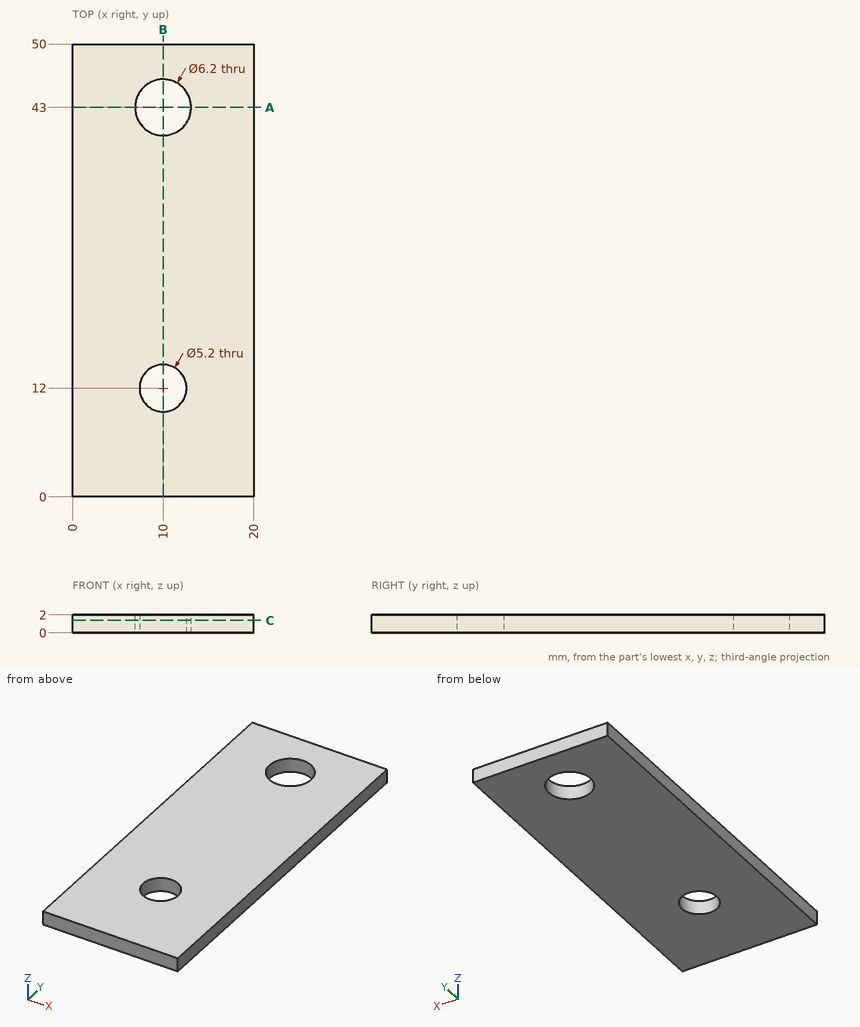
Study the drawing (mm; zero at the part's minimum x, y, z) and answer. Coordinates: 2 decimals unless noted, no trailing zeros. Loops run counter-clockwise (first coordinate to the right, second up) from the corner with the lowest first, then second, coordinate; pieces in that order, holes last. Notation, with made-up numbers: M -31.5,35 L 2.5,35 A22 cw 2.5,70 Z; hole C 54.5,24.25 d11. An arc over 180 degrees is marked long. Answer in a Markdown table with one row per item. Add a question column.
1. Consider L1, parallel to Y at x = 10, z = 0.5; L2, parallel to Y at x = 11.5, z = 0.2; L3, parallel to X at y = 42.5, z = 0.15. Determine where each line is inside the solid, lowest interval first.
2. A flat-ended cylindrical pin translates along its axis: P1, Ø5, axis at x = 10, y = 43, coming from the +Z side. Find the tip coordinate at first contact, or state that the pin passes through.
3. Find section C-C, the plane z = 1.4. Write down the section's boundary in (x, y).
4. Find section A-A, the plane y = 43. Write down the section's boundary in (x, z), then the cut area to 3 significant figures.
5. Find section B-B, the plane x = 10. Write down the section's boundary in (y, z), then the cut area to 3 significant figures.
Reported:
| question | item | result |
|---|---|---|
| 1 | L1 | y = 0 to 9.4, 14.6 to 39.9, 46.1 to 50 |
| 1 | L2 | y = 0 to 9.88, 14.12 to 40.29, 45.71 to 50 |
| 1 | L3 | x = 0 to 6.94, 13.06 to 20 |
| 2 | P1 | passes through |
| 3 | outline | M 0,0 L 20,0 L 20,50 L 0,50 Z; hole C 10,43 d6.2; hole C 10,12 d5.2 |
| 4 | outline | M 0,0 L 6.9,0 L 6.9,2 L 0,2 Z; M 13.1,0 L 20,0 L 20,2 L 13.1,2 Z |
| 4 | area | 27.6 mm^2 |
| 5 | outline | M 0,0 L 9.4,0 L 9.4,2 L 0,2 Z; M 14.6,0 L 39.9,0 L 39.9,2 L 14.6,2 Z; M 46.1,0 L 50,0 L 50,2 L 46.1,2 Z |
| 5 | area | 77.2 mm^2 |
